```python
from build123d import *

# Parameters (mm, degrees)
SKETCH2_R           = 4.445
BOSS_EXTRUDE1_DEPTH = 3.175


with BuildPart() as part:
    # Sketch2 → Boss-Extrude1 (new body)
    with BuildSketch(Plane(origin=(0, 0, 0), x_dir=(0, 0, -1), z_dir=(1, 0, 0))):
        Circle(SKETCH2_R)
        with BuildLine():
            Line((1.905, 3.175), (-1.905, 3.175))
            ThreePointArc((-1.905, 3.175), (-2.803025612, 2.803025612), (-3.175, 1.905))
            Line((-3.175, 1.905), (-3.175, -1.905))
            ThreePointArc((-3.175, -1.905), (-2.803025612, -2.803025612), (-1.905, -3.175))
            Line((-1.905, -3.175), (1.905, -3.175))
            ThreePointArc((1.905, -3.175), (2.803025612, -2.803025612), (3.175, -1.905))
            Line((3.175, -1.905), (3.175, 1.905))
            ThreePointArc((3.175, 1.905), (2.803025612, 2.803025612), (1.905, 3.175))
        make_face(mode=Mode.SUBTRACT)
    extrude(amount=BOSS_EXTRUDE1_DEPTH)


solid = part.part
```
Part model, mm, in its own coordinate system. Round coordinates to 2 decimals unless told otherwise and drop trailing zeros. Write each loop counter-clockwise with the first axis right and the second up, starting at its lowest first coordinate (ties: lowest second). Pieces come first, ordered by that corner, then holes. Notation, with made-up numbers: M 40.5,11.25 L 96.5,11.25 A19 cw 96.5,46.25 Z; hole C 70,48 d2. An arc over 180 degrees is marked long. Answer as CSV lines item,"result". Start each with the question number.
1) Drill centre lines: L1, parallel to Y at x = 2.05, z = 1.5 (3 decimals); L2, parallel to Y at x = 2, z = 0 (3 decimals); L3, parallel to Z at x = 2.65, y = 2.5. Where is each one in solid material? Low to high.
2) Drop flat-ended pins along their axis: pin 1 (2 mm diameter, centred on y = -1, z = 0.5, fed in from +X); pin 2 (1 mm diameter, centred on x = 2, z = 3, fed in from -Y). Give the stop position or say it passes through.
3) Mould opens along Z. For faces 1 (the face through (1.57, -4.34, 0.96)), 2 (the face through (2, -3.175, 0)) say: +Z half, -Z half, draft (parallel to the pull), parting line (faces both ways), or undercut.
4) Band-saw the part on C-C (x = 2.6). List the corners of the cut face in (y, z) (3 decimals), then the cut area to 3 significant figures.
5) Band-saw the part on A-A (y = 0). List the corners of the cut face in (x, z) (3 decimals).
6) Band-saw the part on D-D (y = 4.25). List the corners of the cut face in (x, z) (3 decimals).
Worked out:
1,L1,"-4.184 to -3.175, 3.175 to 4.184"
1,L2,"-4.445 to -3.175, 3.175 to 4.445"
1,L3,"-3.68 to -3.03, 3.03 to 3.68"
2,pin 1,"through"
2,pin 2,"y = -3.68"
3,face 1,"parting line"
3,face 2,"undercut"
4,outline,"C 0,0 d8.89; hole M -3.175,-1.905 A1.27 ccw -1.905,-3.175 L 1.905,-3.175 A1.27 ccw 3.175,-1.905 L 3.175,1.905 A1.27 ccw 1.905,3.175 L -1.905,3.175 A1.27 ccw -3.175,1.905 Z"
4,area,"23.1 mm²"
5,outline,"M 0,-4.445 L 3.175,-4.445 L 3.175,-3.175 L 0,-3.175 Z; M 0,3.175 L 3.175,3.175 L 3.175,4.445 L 0,4.445 Z"
6,outline,"M 0,-1.302 L 3.175,-1.302 L 3.175,1.302 L 0,1.302 Z"
